from build123d import *

# Parameters (mm, degrees)
F2_W     = 8
F2_H     = 16
F3_DEPTH = 77.17437
F4_R     = 1.25
F5_DEPTH = 2


with BuildPart() as f1:
    # F0 (on Front) → F1 (revolve)
    with BuildSketch(Plane.XZ):
        Polygon((43.25, 0), (35.25, 0), (35.25, -49.948681), (66.444077, -130), (69.693929, -130), (38.25, -49.3075), (38.25, -2.400862), (43.25, -2.400862), align=None)
    revolve(axis=Axis((0, 0, -40), (0, 0, -1)))

    # F2 (on Right) → F3 (cut)
    with BuildSketch(Plane.YZ):
        with Locations((-4, -110)):
            Rectangle(F2_W, F2_H)
        with Locations((4, -110)):
            Rectangle(F2_W, F2_H)
    extrude(amount=F3_DEPTH, mode=Mode.SUBTRACT)

    # F4 (on face) → F5 (join)
    with BuildSketch(Plane.XY):
        with Locations((0, 39.2)):
            Circle(F4_R)
        with Locations((-39.2, 0)):
            Circle(F4_R)
        with Locations((0, -39.2)):
            Circle(F4_R)
        with Locations((39.2, 0)):
            Circle(F4_R)
    extrude(amount=F5_DEPTH)


solid = f1.part
Work out the finished part from the listing and answer in its coordinate system (mm). A direction names the side the tool comes from. Coordinates: 2 decimals unless noted, no trailing zeros. Write each loop counter-clockwise with the first axis right and the second up, starting at its lowest first coordinate (ties: lowest second). Pieces come first, ordered by that corner, then holes. Notation, with made-up numbers: M 10.5,78 L 19.5,78 A18 cw 19.5,83 Z; hole C 7,64 d11. An arc over 180 degrees is marked long. Use one line per item in the form item = value. Start each with the question number.
1. Each of these flat-tipped pins is pushed along its axis until it touches: P1, Ø4, axis at y = -39.5, z = -91, coming from the -X side; P2, Ø4, axis at x = 62.5, y = -3, coming from the +Z side; P3, Ø8, axis at x = 15.5, z = -82, coming from the -Y side. Where does it stop, or does it pass through?
2. Straight lines are drawn through the part: probe 1 along Y at (x, z) = (0, -22); probe 2 along Y at (x, z) = (21, -100.5). For each, find the intervals that lie inside material, in ascending order. Write a range as from..to.
3. A tool of negligible diameter and unlimited length cuts with its end or side. For faces 1 (the face through (57, 0, -102)), 2 (the face through (-30.354, 23.275, -25.526)), 3 (the face through (-34.32, 26.32, -1.18)), 4 (the face through (60, -8, -110)), from which of +Z, -Z, +X, -X, +Y, -Y can it reach the whole face along a straight path? Write none if from no direction.
4. The part is cut by section B-B (z = -95.5). Give the vertices of the cut face in (x, y).
5. The part is cut by section A-A (z = -30.5). Give the vertices of the cut face in (x, y), plus the area to 3 significant figures.
6. The mould has two halves that part along X. Classify faces 5 (the face through (21.58, 41.49, -71.16)), 6 (the face through (42.095, -13.256, -72.746)), 7 (the face through (-16, 35, -2.401)): released by +X, released by -X, zero draft, split by the parting line, or undercut.
Evaluation:
q1.P1 = -39.83
q1.P2 = -118
q1.P3 = -50.57
q2.probe_1 = -38.25..-35.25, 35.25..38.25
q2.probe_2 = -54.28..-50.78, 50.78..54.28
q3.face_1 = -Z, +X
q3.face_2 = none
q3.face_3 = +Z
q3.face_4 = +X
q4.outline = C 0,0 d112.5; hole C 0,0 d106
q5.outline = C 0,0 d76.5; hole C 0,0 d70.5
q5.area = 693 mm^2
q6.face_5 = split by the parting line
q6.face_6 = undercut
q6.face_7 = zero draft
